Work out the finished part from the listing and answer in its coordinate system (mm). Face numbers are marked on the shaded views. A direction names the side the tool comes from. Give positions to 0.01 mm unless a question says otherwise; leave off trailing zeros. Order: outer loops, then holes, each group sorted by start corner. A loop starts at its lowest first (then second) coordinate and runs counter-clockwise, first axis right, second up. Notation, with made-up numbers: (35.25, 42.5) - (65.25, 42.5) arc R27 ccw to (65.25, 62.5) - close; hole circle Ø6 at (2.25, 55). An arc over 180 degrees is marked (long way). Write each question's results on one line, items separated by ' | '.
from build123d import *

# Parameters (mm, degrees)
F0_R         = 3.5
F1_DEPTH     = 28
F2_W         = 28
F2_H         = 27.9113203287
F2_R         = 1.4
F3_DEPTH     = 5
F4_R         = 2.5
F5_T1_DEPTH  = 17.5
F5_T4_ANGLE  = 90
F5_T6_ANGLE  = 90
F5_T8_ANGLE  = 90
F5_T10_ANGLE = 90
F0_R_2       = 1.25
F6_DEPTH     = 10


# Not quite as in the source:
# - a fillet or chamfer that OpenCascade refuses, or shapes differently, is made with other operations: its cross-section is extruded or revolved along the edge and cut away or added


with BuildPart() as f1:
    # F0 (on Front) → F1 (new body)
    with BuildSketch(Plane.XZ):
        with BuildLine():
            Line((3.528, 5.0124127732), (-3.528, 5.0124127732))
            ThreePointArc((-3.528, 5.0124127732), (-4.7310778559, 3.8971743778), (-5.5952764673, 2.5027878582))
            Line((-5.5952764673, 2.5027878582), (-7.5016845949, 2.5027878582))
            Line((-7.5016845949, 2.5027878582), (-7.5016845949, -2.5444291532))
            Line((-7.5016845949, -2.5444291532), (-5.5764635831, -2.5444291532))
            ThreePointArc((-5.5764635831, -2.5444291532), (0, -6.1295241095), (5.5764635831, -2.5444291532))
            Line((5.5764635831, -2.5444291532), (7.4870199896, -2.5444291532))
            Line((7.4870199896, -2.5444291532), (7.4870199896, 2.5027878582))
            Line((7.4870199896, 2.5027878582), (5.5952764673, 2.5027878582))
            ThreePointArc((5.5952764673, 2.5027878582), (4.7310778559, 3.8971743778), (3.528, 5.0124127732))
        make_face()
        Circle(F0_R, mode=Mode.SUBTRACT)
    extrude(amount=F1_DEPTH)

    # F2 (on Front) → F3 (join)
    with BuildSketch(Plane.XZ):
        Rectangle(F2_W, F2_H)
        with Locations((-7.7399509028, -7.7685024589)):
            Circle(F2_R, mode=Mode.SUBTRACT)
        with Locations((7.8511200845, 7.7744480222)):
            Circle(F2_R, mode=Mode.SUBTRACT)
    extrude(amount=F3_DEPTH)

    # F4
    f4_edges = [f1.edges().sort_by_distance(p)[0] for p in [
        (14, 0, 0),
        (0, 0, -13.95566),
        (-14, 0, 0),
        (0, 0, 13.95566),
    ]]
    fillet(f4_edges, radius=F4_R)

    # F5: fillet of radius 5 on 4 edges, made by hand

    # F5_s2 → F5_t1 (cut)
    with BuildSketch(Plane.XZ):
        with BuildLine():
            ThreePointArc((-9, 13.9556601644), (-12.5355339059, 12.4911940703), (-14, 8.9556601644))
            Line((-14, 8.9556601644), (-14, 13.9556601644))
            Line((-14, 13.9556601644), (-9, 13.9556601644))
        make_face()
        with BuildLine():
            ThreePointArc((14, 8.9556601644), (12.5355339059, 12.4911940703), (9, 13.9556601644))
            Line((9, 13.9556601644), (14, 13.9556601644))
            Line((14, 13.9556601644), (14, 8.9556601644))
        make_face()
        with BuildLine():
            ThreePointArc((14, -8.9556601644), (12.5355339059, -12.4911940703), (9, -13.9556601644))
            Line((9, -13.9556601644), (14, -13.9556601644))
            Line((14, -13.9556601644), (14, -8.9556601644))
        make_face()
        with BuildLine():
            ThreePointArc((-9, -13.9556601644), (-12.5355339059, -12.4911940703), (-14, -8.9556601644))
            Line((-14, -8.9556601644), (-14, -13.9556601644))
            Line((-14, -13.9556601644), (-9, -13.9556601644))
        make_face()
    extrude(amount=F5_T1_DEPTH, mode=Mode.SUBTRACT)

    # F5_s3 → F5_t4 (revolve, cut)
    with BuildSketch(Plane.YZ.offset(-9)):
        with BuildLine():
            ThreePointArc((0, -11.4556601644), (-0.732233047, -13.2234271173), (-2.5, -13.9556601644))
            Line((-2.5, -13.9556601644), (0, -13.9556601644))
            Line((0, -13.9556601644), (0, -11.4556601644))
        make_face()
    revolve(axis=Axis((-9, 0, -8.9556601644), (0, 1, 0)), revolution_arc=F5_T4_ANGLE, mode=Mode.SUBTRACT)

    # F5_s5 → F5_t6 (revolve, cut)
    with BuildSketch(Plane.XY.offset(-8.9556601644)):
        with BuildLine():
            ThreePointArc((11.5, 0), (13.267766953, -0.732233047), (14, -2.5))
            Line((14, -2.5), (14, 0))
            Line((14, 0), (11.5, 0))
        make_face()
    revolve(axis=Axis((9, 0, -8.9556601644), (0, 1, 0)), revolution_arc=F5_T6_ANGLE, mode=Mode.SUBTRACT)

    # F5_s7 → F5_t8 (revolve, cut)
    with BuildSketch(Plane.YZ.offset(9)):
        with BuildLine():
            ThreePointArc((0, 11.4556601644), (-0.732233047, 13.2234271173), (-2.5, 13.9556601644))
            Line((-2.5, 13.9556601644), (0, 13.9556601644))
            Line((0, 13.9556601644), (0, 11.4556601644))
        make_face()
    revolve(axis=Axis((9, 0, 8.9556601644), (0, 1, 0)), revolution_arc=F5_T8_ANGLE, mode=Mode.SUBTRACT)

    # F5_s9 → F5_t10 (revolve, cut)
    with BuildSketch(Plane.XY.offset(8.9556601644)):
        with BuildLine():
            ThreePointArc((-11.5, 0), (-13.267766953, -0.732233047), (-14, -2.5))
            Line((-14, -2.5), (-14, 0))
            Line((-14, 0), (-11.5, 0))
        make_face()
    revolve(axis=Axis((-9, 0, 8.9556601644), (0, 1, 0)), revolution_arc=F5_T10_ANGLE, mode=Mode.SUBTRACT)

    # F0 (on Front) → F6 (cut)
    with BuildSketch(Plane.XZ):
        Circle(F0_R_2)
    extrude(amount=F6_DEPTH, mode=Mode.SUBTRACT)


solid = f1.part
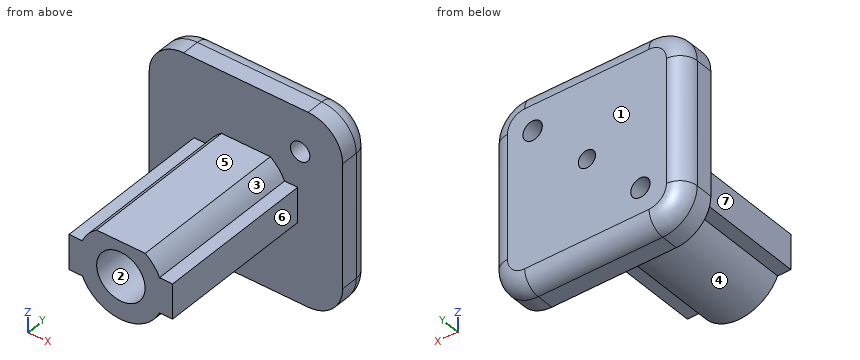
1. A cutting plane is placed at A-A, the plane z = 0. Write down the section's boundary in (x, y), then the cut area to 3 significant figures.
Answer list:
outline: (-14, -5) - (-7.5, -5) - (-7.5, -28) - (-3.5, -28) - (-3.5, -5) - (-1.25, -5) - (-1.25, 0) - (-11.5, 0) arc R2.5 ccw to (-14, -2.5) - close; (1.25, -5) - (3.5, -5) - (3.5, -28) - (7.49, -28) - (7.49, -5) - (14, -5) - (14, -2.5) arc R2.5 ccw to (11.5, 0) - (1.25, 0) - close | area: 309 mm^2
2. Given P1, Ø2, axis at x = -7.74, z = -7.77, coming from the -Y side; P2, Ø1, axis at x = -6.5, z = -8.5, coming from the -Y side; P3, Ø0.6, axis at x = 7, y = -19.5, coming from the +Z side; P4, Ø5, axis at y = -15, z = -4.5, coming from the -X side, each flat-ended and moving along its own axis, determine where each tip first touches the part or whether it passes through.
Answer list:
P1: through | P2: y = -5 | P3: z = 2.5 | P4: x = -7.5
3. A cutting plane is placed at C-C, the plane y = -22. Write down the section's boundary in (x, z).
Answer list:
outline: (-7.5, -2.54) - (-5.58, -2.54) arc R6.13 ccw to (5.58, -2.54) - (7.49, -2.54) - (7.49, 2.5) - (5.6, 2.5) arc R6.13 ccw to (3.53, 5.01) - (-3.53, 5.01) arc R6.13 ccw to (-5.6, 2.5) - (-7.5, 2.5) - close; hole circle Ø7 at (0, 0)
4. Straight lines are drawn through the part: line 1 (Z direction, x = 0.25, y = -6); line 2 (Z direction, x = 0, y = -3.9); line 3 (X direction, y = -10, z = 0). For each, find the intervals that lie inside material, in ascending order. Write a range as [from, to].
Answer list:
line 1: [-6.12, -3.49], [3.49, 5.01] | line 2: [-13.96, -1.25], [1.25, 13.96] | line 3: [-7.5, -3.5], [3.5, 7.49]
5. A cutting plane is placed at D-D, the plane x = 5. Write down the section's boundary in (y, z).
Answer list:
outline: (-28, -3.55) - (-5, -3.55) - (-5, -13.96) - (-2.5, -13.96) arc R2.5 ccw to (0, -11.46) - (0, 11.46) arc R2.5 ccw to (-2.5, 13.96) - (-5, 13.96) - (-5, 3.55) - (-28, 3.55) - close
6. Determine the mould class of the marked faces 1, 2 and 3 for opening direction X: +X half, -X half, draft (parallel to the pull), parting line (faces both ways), or undercut.
Answer list:
face 1: draft | face 2: undercut | face 3: +X half
7. A tool of negligible diameter and unlimited length cuts with its end or side. For the marked faces 4, 5, 6 and 7, from which of +Z, -Z, +X, -X, +Y, -Y can it reach the whole face along a straight path? Write none if from no direction.
Answer list:
face 4: -Z, -Y | face 5: +Z, +X, -X, -Y | face 6: +Z, -Z, +X, -Y | face 7: +Z, -Z, -X, -Y
8. A cutting plane is placed at B-B, the plane x = 0. Write down the section's boundary in (y, z), then the cut area to 3 significant figures.
Answer list:
outline: (-28, -6.13) - (-5, -6.13) - (-5, -13.96) - (-2.5, -13.96) arc R2.5 ccw to (0, -11.46) - (0, -1.25) - (-5, -1.25) - (-5, -3.5) - (-28, -3.5) - close; (-28, 3.5) - (-5, 3.5) - (-5, 1.25) - (0, 1.25) - (0, 11.46) arc R2.5 ccw to (-2.5, 13.96) - (-5, 13.96) - (-5, 5.01) - (-28, 5.01) - close | area: 220 mm^2
